The listing builds one solid part. Answer for the finished solid, in the listing's coordinates (mm). Face numbers are marked on the shaded views. Round coordinates to 2 decimals unless told otherwise and drop trailing zeros. Write each loop counter-clockwise with the first axis right and the second up, starting at its lowest first coordinate (ties: lowest second). Pieces come first, ordered by that corner, then holes. Notation, with made-up numbers: M -19.75,16.5 L 23.25,16.5 A16 ccw 23.25,27.5 Z; hole C 31,16 d3. An arc over 180 degrees is marked long. Write each question's results on one line, items separated by ' | '.
from build123d import *

# Parameters (mm, degrees)
SKETCH_1_R          = 51
EXTRUDE_1_DEPTH     = 1
SKETCH_2_R          = 1.5
CUT_EXTRUDE_1_DEPTH = 73.131823767
SKETCH_3_W          = 3
SKETCH_3_H          = 1
CUT_EXTRUDE_2_DEPTH = 73.131823767


with BuildPart() as part:
    # 草图1 → 凸台-拉伸1 (new body)
    with BuildSketch(Plane(origin=(0, 0, 0), x_dir=(1, 0, 0), z_dir=(0, 1, 0))):
        with Locations(Location((0, 0, 0), (0, 0, 270))):
            Circle(SKETCH_1_R)
    extrude(amount=EXTRUDE_1_DEPTH)

    # 草图2 → 切除-拉伸1 (cut, through all)
    with BuildSketch(Plane(origin=(0, 1, 0), x_dir=(1, 0, 0), z_dir=(0, 1, 0))):
        with Locations((0, 50.5)):
            Circle(SKETCH_2_R)
        with Locations((-43.734282891, -25.25)):
            Circle(SKETCH_2_R)
        with Locations((43.734282891, -25.25)):
            Circle(SKETCH_2_R)
    extrude(amount=-CUT_EXTRUDE_1_DEPTH, mode=Mode.SUBTRACT)

    # 草图3 → 切除-拉伸2 (cut, through all)
    with BuildSketch(Plane(origin=(0, 1, 0), x_dir=(1, 0, 0), z_dir=(0, 1, 0))):
        Polygon((-44.484282891, -23.950961894), (-45.350308295, -24.450961894), (-43.850308295, -27.049038106), (-42.984282891, -26.549038106), align=None)
        with Locations((0, 51)):
            Rectangle(SKETCH_3_W, SKETCH_3_H)
        Polygon((44.484282891, -23.950961894), (42.984282891, -26.549038106), (43.850308295, -27.049038106), (45.350308295, -24.450961894), align=None)
    extrude(amount=-CUT_EXTRUDE_2_DEPTH, mode=Mode.SUBTRACT)


solid = part.part
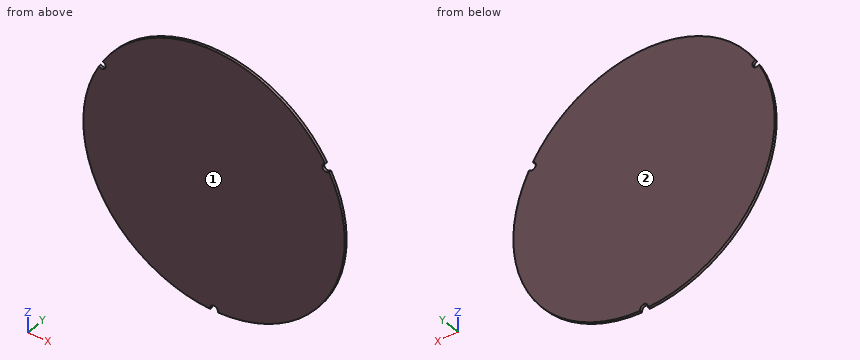
1) The mould has two halves that part along Y. Classify the marked faces 1 and 2: +Y half, -Y half, draft (parallel to the pull), parting line (faces both ways), or undercut.
Return value:
face 1: -Y half | face 2: +Y half
2) Section A-A (y = 0.5) is taken. Determine the outline of the cut face in (x, z).
Return value:
outline: M -44.9,24.19 A51 ccw -1.5,-50.98 L -1.5,-50.5 A1.5 cw 1.5,-50.5 L 1.5,-50.98 A51 ccw 44.9,24.19 L 44.48,23.95 A1.5 cw 42.98,26.55 L 43.4,26.79 A51 ccw -43.4,26.79 L -42.98,26.55 A1.5 cw -44.48,23.95 Z
3) This flat-tipped pin is pushed along its axis until it touches: pin 1 (1.5 mm diameter, centred on x = -6, z = -25, fed in from -Y). Where does it stop, or does it pass through?
Return value:
pin 1: y = 0
4) Section C-C (z = -24) is taken. Determine the outline of the cut face in (x, y), then the cut area to 3 significant figures.
Return value:
outline: M -45,0 L 45,0 L 45,1 L -45,1 Z | area: 90.0 mm²
5) Section B-B (x = 0) is taken. Determine the outline of the cut face in (y, z), then the cut area to 3 significant figures.
Return value:
outline: M 0,-49 L 1,-49 L 1,51 L 0,51 Z | area: 100 mm²
6) Find the intervals of material crossed by line 1 (X direction, y = 0.45, z = 24); line 2 (Z direction, x = 34, y = 0.7); line 3 (Z direction, x = 40.5, y = 0.45), in increasing order.
Return value:
line 1: -45 to -44.57, -42.91 to 42.91, 44.57 to 45 | line 2: -38.01 to 38.01 | line 3: -31 to 31
